from build123d import *

# Parameters (mm, degrees)
F1_DEPTH = 15
F2_R     = 53.5
F3_DEPTH = 20
F4_R     = 52.5
F5_DEPTH = 16
F6_R     = 10
F7_DEPTH = 11


with BuildPart() as f1:
    # F0 (on Front) → F1 (new body)
    with BuildSketch(Plane.XZ):
        with BuildLine():
            Line((67, -23.49468), (67, 23.49468))
            ThreePointArc((67, 23.49468), (-71, 0), (67, -23.49468))
        make_face()
    extrude(amount=F1_DEPTH)

    # F2 (on face) → F3 (join)
    with BuildSketch(Plane.XZ.offset(15)):
        Circle(F2_R)
    extrude(amount=F3_DEPTH)

    # F4 (on face) → F5 (join)
    with BuildSketch(Plane.XZ.offset(35)):
        Circle(F4_R)
    extrude(amount=F5_DEPTH)

    # F6 (on face) → F7 (cut)
    with BuildSketch(Plane.XZ.offset(51)):
        with Locations((10.5, -10.5)):
            Circle(F6_R)
    extrude(amount=-F7_DEPTH, mode=Mode.SUBTRACT)


solid = f1.part
Input: part model. Units: mm. Frame: model coordinates. A direction names the side the tool comes from. Give positions to 0.01 mm unless a question says otherwise; leave off trailing zeros. Loops run counter-clockwise (first coordinate to the right, second up) from the corner with the lowest first, then second, coordinate; pieces in that order, holes last. Notation, with made-up numbers: (74.5, 38.5) -> (88.5, 38.5) arc R15 ccw to (88.5, 44.5) -> close; hole circle Ø10 at (65.25, -29). An arc over 180 degrees is marked (long way). Answer as a JSON object with one key per item and string values. Group by question number.
Item 1: Cut plane C-C, the plane y = -22.5. Return the cut outline in (x, z).
Item 2: Cut plane A-A, the plane z = 48. Return the cut outline in (x, y), and give its area (3 significant figures).
Item 3: Cut plane B-B, the plane x = -17.5. Return the cut outline in (y, z), and give its area (3 significant figures).
Item 4: Reachability of faces 1 (the cylindrical face through (-70.945, -7.395, 2.787)), 2 (the cylindrical face through (50.076, -42.888, 15.77)) from +Z, -Z, +X, -X, +Y, -Y: full face, straight path, thin tool, end or side. Return the list, or none.
Item 5: Line query: probe 1 along Y at (x, z) = (-60.5, -1); probe 2 along Z at (x, y) = (10, -42); probe 3 along X at (y, z) = (-23, -5.5). Output: solid intervals per line, ascending.
Item 6: Cut plane D-D, the plane z = -10.5. Return the cut outline in (x, y), and give its area (3 significant figures).
Item 7: Pin query (flat end, axial travel): P1, Ø5, axis at y = -22, z = 17.5, coming from the -X side; P2, Ø12, axis at x = 10.5, z = -10.5, coming from the +Y side; P3, Ø10, axis at y = -32, z = 40.5, coming from the -X side (3 decimals); P4, Ø1, axis at x = 12.5, z = -52, coming from the -Y side. Return the tip coordinate at first contact, or that it passes through.
Checks:
{
 "1": {"outline": "circle Ø107 at (0, 0)"},
 "2": {"outline": "(-52.32, -15) -> (-23.63, -15) -> (-23.63, -35) -> (-21.27, -35) -> (-21.27, -51) -> (21.27, -51) -> (21.27, -35) -> (23.63, -35) -> (23.63, -15) -> (52.32, -15) -> (52.32, 0) -> (-52.32, 0) -> close", "area": "3,200 mm²"},
 "3": {"outline": "(-51, -49.5) -> (-35, -49.5) -> (-35, -50.56) -> (-15, -50.56) -> (-15, -68.81) -> (0, -68.81) -> (0, 68.81) -> (-15, 68.81) -> (-15, 50.56) -> (-35, 50.56) -> (-35, 49.5) -> (-51, 49.5) -> close", "area": "5,670 mm²"},
 "4": {"face 1": "+Y, -Y", "face 2": "-Y"},
 "5": {"probe 1": "y = -15 to 0", "probe 2": "z = -51.54 to -20.49, -0.51 to 51.54", "probe 3": "x = -53.22 to 53.22"},
 "6": {"outline": "(-70.22, -15) -> (-52.46, -15) -> (-52.46, -35) -> (-51.44, -35) -> (-51.44, -51) -> (0.5, -51) -> (0.5, -40) -> (20.5, -40) -> (20.5, -51) -> (51.44, -51) -> (51.44, -35) -> (52.46, -35) -> (52.46, -15) -> (67, -15) -> (67, 0) -> (-70.22, 0) -> close", "area": "5,580 mm²"},
 "7": {"P1": "stops at x = -51.35", "P2": "stops at y = 0", "P3": "stops at x = -40.025", "P4": "stops at y = -35"}
}
